```python
from build123d import *

# Parameters (mm, degrees)
SKETCH1_W           = 150
SKETCH1_H           = 150
BOSS_EXTRUDE1_DEPTH = 10
SKETCH2_R           = 15
SKETCH2_R_2         = 16
CUT_EXTRUDE1_DEPTH  = 25


with BuildPart() as part:
    # Sketch1 → Boss-Extrude1 (new body)
    with BuildSketch(Plane(origin=(0, 0, 0), x_dir=(0, 0, -1), z_dir=(1, 0, 0))):
        Rectangle(SKETCH1_W, SKETCH1_H)
    extrude(amount=BOSS_EXTRUDE1_DEPTH)

    # Sketch2 → Cut-Extrude1 (cut)
    with BuildSketch(Plane(origin=(10, 0, 0), x_dir=(0, 0, -1), z_dir=(1, 0, 0))):
        Circle(SKETCH2_R)
        with Locations((0, 38.727703316)):
            Circle(SKETCH2_R_2)
        with Locations((33.539174902, 19.363851658)):
            Circle(SKETCH2_R_2)
        with Locations((33.539174902, -19.363851658)):
            Circle(SKETCH2_R_2)
        with Locations((0, -38.727703316)):
            Circle(SKETCH2_R_2)
        with Locations((-33.539174902, -19.363851658)):
            Circle(SKETCH2_R_2)
        with Locations((-33.539174902, 19.363851658)):
            Circle(SKETCH2_R_2)
    extrude(amount=-CUT_EXTRUDE1_DEPTH, mode=Mode.SUBTRACT)


solid = part.part
```
Source: CAD feature listing. Evaluate the final solid. Frame: model axes, mm. Round coordinates to 2 decimals unless told otherwise and drop trailing zeros. Write each loop counter-clockwise with the first axis right and the second up, starting at its lowest first coordinate (ties: lowest second). Pieces come first, ordered by that corner, then holes. Notation, with made-up numbers: M 58.5,73.5 L 75.5,73.5 A16 cw 75.5,92.5 Z; hole C 35,-11.5 d5. An arc over 180 degrees is marked long. Answer as a JSON object with one key per item and string values. Group by question number.
(1) Section query B-B on z = 0. Output: boundary loops of the cut face in (x, y), then the cut area to 3 significant figures.
(2) Section query D-D on x = 3.75. Output: boundary loops of the cut face in (y, z).
(3) Ray query, line 1 (Z direction, x = 7, y = 32); line 2 (Z direction, x = 1.75, y = -39); line 3 (Y direction, x = 2, z = -38). Return the intervals inside material, ascending. Write a range as [from, to].
(4) Section query C-C on z = 39.5. Output: boundary loops of the cut face in (x, y), then the cut area to 3 significant figures.
(5) Mould query, pull axis Y, two halves, no side actions, for faces 1 (the cylindrical face through (5.07, 0.66, 14.985)), 2 (the flat face through (0, 1, 18)), 3 (the flat face through (5, 75, 1)). Classes: +Y half, -Y half, draft (parallel to the pull), parting line (faces both ways), or undercut.
(6) Section query A-A on y = 0. Output: boundary loops of the cut face in (x, z).
Computed values:
{
 "1": {"outline": "M 0,-75 L 10,-75 L 10,-54.73 L 0,-54.73 Z; M 0,-22.73 L 10,-22.73 L 10,-15 L 0,-15 Z; M 0,15 L 10,15 L 10,22.73 L 0,22.73 Z; M 0,54.73 L 10,54.73 L 10,75 L 0,75 Z", "area": "560 mm^2"},
 "2": {"outline": "M -75,-75 L 75,-75 L 75,75 L -75,75 Z; hole C -38.73,0 d32; hole C -19.36,-33.54 d32; hole C -19.36,33.54 d32; hole C 0,0 d30; hole C 19.36,-33.54 d32; hole C 19.36,33.54 d32; hole C 38.73,0 d32"},
 "3": {"line 1": "[-75, -43.35], [-23.72, -14.52], [14.52, 23.72], [43.35, 75]", "line 2": "[-75, -16], [16, 75]", "line 3": "[-75, -34.73], [-4, 4], [34.73, 75]"},
 "4": {"outline": "M 0,-75 L 10,-75 L 10,-34.21 L 0,-34.21 Z; M 0,-4.52 L 10,-4.52 L 10,4.52 L 0,4.52 Z; M 0,34.21 L 10,34.21 L 10,75 L 0,75 Z", "area": "906 mm^2"},
 "5": {"face 1": "undercut", "face 2": "draft", "face 3": "+Y half"},
 "6": {"outline": "M 0,-75 L 10,-75 L 10,-15 L 0,-15 Z; M 0,15 L 10,15 L 10,75 L 0,75 Z"}
}
